```python
from build123d import *

# Parameters (mm, degrees)
SKETCH_1_R            = 75
EXTRUDE_1_DEPTH       = 15
SKETCH_2_R            = 10
CUT_EXTRUDE_2_DEPTH   = 10
FILLET_1_R            = 2
CHAMFER_1_SIZE        = 1
SKETCH_3_R            = 6.5
CUT_EXTRUDE_3_DEPTH   = 2
CUT_EXTRUDE_START     = 69.96131425
CUT_EXTRUDE_9_DEPTH   = 6.03868575
CUT_EXTRUDE_START_2   = 5
CUT_EXTRUDE_9_2_DEPTH = 6


with BuildPart() as part:
    # 草图1 → 凸台-拉伸1 (new body)
    with BuildSketch(Plane(origin=(0, 0, 0), x_dir=(1, 0, 0), z_dir=(0, 1, 0))):
        with Locations(Location((0, 0, 0), (0, 0, 270))):
            Circle(SKETCH_1_R)
    extrude(amount=EXTRUDE_1_DEPTH)

    # 草图2 → 切除-拉伸2 (cut)
    with BuildSketch(Plane(origin=(0, 0, 0), x_dir=(1, 0, 0), z_dir=(0, 1, 0))):
        with Locations(Location((-35, 0, 0), (0, 0, 270))):
            Circle(SKETCH_2_R)
    extrude(amount=CUT_EXTRUDE_2_DEPTH, mode=Mode.SUBTRACT)

    # 圆角1
    fillet_1_edges = [part.edges().sort_by_distance(p)[0] for p in [
        (0, 0, -75),
    ]]
    fillet(fillet_1_edges, radius=FILLET_1_R)

    # 倒角1
    chamfer_1_edges = [part.edges().sort_by_distance(p)[0] for p in [
        (-35, 0, -10),
    ]]
    chamfer(chamfer_1_edges, length=CHAMFER_1_SIZE)

    # 草图3 → 切除-拉伸3 (cut)
    with BuildSketch(Plane.XZ):
        with Locations(Location((30, 0, 0), (0, 0, 270))):
            Circle(SKETCH_3_R)
    extrude(amount=-CUT_EXTRUDE_3_DEPTH, mode=Mode.SUBTRACT)

    # 切除-拉伸9: read off the stored shape, not the designer's step
    # 切除-拉伸9 outline → 切除-拉伸9 (cut)
    with BuildSketch(Plane(origin=(0, 0, 0), x_dir=(0, 0, -1), z_dir=(1, 0, 0)).offset(CUT_EXTRUDE_START)):
        with BuildLine():
            add(Edge.make_bspline(
                [(-2.408599358, 7.908599358), (-2.408599358, 7.380050553), (-2.19172637, 6.863241712), (-1.453678928, 6.125309354), (-0.931504849, 5.908902276), (0.111986372, 5.908297113), (0.631291702, 6.120458395), (1.378441313, 6.866818593), (1.591215997, 7.385801707), (1.591585037, 8.429983307), (1.375428682, 8.952297025), (0.638483078, 9.690642916), (0.120902782, 9.908088408), (-0.93423459, 9.909108439), (-1.452163157, 9.692883252), (-2.191245952, 8.954957584), (-2.408599358, 8.437148163), (-2.408599358, 7.908599358)],
                knots=[0, 0, 0, 0, 0.125, 0.125, 0.25, 0.25, 0.375, 0.375, 0.5, 0.5, 0.625, 0.625, 0.75, 0.75, 0.875, 0.875, 1, 1, 1, 1], degree=3))
        make_face()
    extrude(amount=CUT_EXTRUDE_9_DEPTH, mode=Mode.SUBTRACT)

    # Cut-Extrude 9 2 outline → Cut-Extrude 9 2 (add)
    with BuildSketch(Plane(origin=(0, 0, 0), x_dir=(1, 0, 0), z_dir=(0, 1, 0)).offset(CUT_EXTRUDE_START_2)):
        with BuildLine():
            ThreePointArc((69.96131435, -2.408599358), (69.998905417, -0.405199028), (69.982963585, 1.598490525))
            Line((69.982963585, 1.598490525), (69.96131425, 2.614030645))
            Line((69.96131425, 2.614030645), (69.96131435, -2.408599358))
        make_face()
    extrude(amount=CUT_EXTRUDE_9_2_DEPTH)


solid = part.part
```
The model under review builds one solid part; all positions refer to its coordinate system, in mm. A direction names the side the tool comes from. Round coordinates to 2 decimals unless told otherwise and drop trailing zeros. Loops run counter-clockwise (first coordinate to the right, second up) from the corner with the lowest first, then second, coordinate; pieces in that order, holes last. Notation, with made-up numbers: (82.5, 86.5) -> (117.5, 86.5) arc R23 ccw to (117.5, 124.5) -> close; hole circle Ø7 at (43, 32.5). An arc over 180 degrees is marked (long way). Answer in a Markdown table with one row per item.
1) Tool access review of faces 1 (the cylindrical face through (70, 8, 0)), 2 (the flat face through (30, 2, 0)), 3 (the flat face through (1, 15, -1)): name each direction out of +Z, -Z, +X, -X, +Y, -Y from which nothing blocks a thin tool from reaching the whole face with its end or side.
Taken from the geometry:
| item | result |
|---|---|
| face 1 | +X |
| face 2 | -Y |
| face 3 | +Z, -Z, +X, -X, +Y |
2) Wall thickness on line 1 along X through (y, z) = (4, 0); line 2 along X through (y, z) = (1.3, 0); line 3 along X through (y, z) = (5.25, -1): over which ranges is each line inside the solid? List them lowest first.
Taken from the geometry:
| item | result |
|---|---|
| line 1 | x = -75 to -45, -25 to 75 |
| line 2 | x = -74.87 to -45, -25 to 23.5, 36.5 to 74.87 |
| line 3 | x = -74.99 to -44.95, -25.05 to 74.99 |
3) For pin 1 Ø10 at (x, z) = (-38, -0.5) entering from -Y; pin 2 Ø1 at (x, z) = (35.5, -41.5) entering from -Y; pin 3 Ø5 at (y, z) = (10, 5) entering from -X; pin 4 Ø2 at (x, y) = (-15.5, 12.5) entering from +Z (3 decimals), all flat-tipped, find the tip position at first contact; note any pin that passes through.
Taken from the geometry:
| item | result |
|---|---|
| pin 1 | stops at y = 10 |
| pin 2 | stops at y = 0 |
| pin 3 | stops at x = -74.96 |
| pin 4 | stops at z = 73.585 |
4) Draft analysis for pull direction X (two halves, no side actions). For faces 4 (the cylindrical face through (-45.636, 8.409, -59.517)), 5 (the cylindrical face through (-44.76, 5.44, -2.17)), 6 (the flat face through (1, 0, -1)), state which applies: pulls with the +X half, pulls with the -X half, needs draft (parallel to the pull), parting line crosses it, or undercut.
Taken from the geometry:
| item | result |
|---|---|
| face 4 | parting line crosses it |
| face 5 | undercut |
| face 6 | needs draft |
5) Consider section A-A, the plane y = 3.75. Write out the cut boundary in (x, z).
Taken from the geometry:
| item | result |
|---|---|
| outline | circle Ø150 at (0, 0); hole circle Ø20 at (-35, 0) |
6) Consider section B-B, the plane y = 12.25. Write out the cut boundary in (x, z), plus the area to 3 significant figures.
Taken from the geometry:
| item | result |
|---|---|
| outline | circle Ø150 at (0, 0) |
| area | 17,700 mm² |
